Can you work these out from the model? Positions are in its coordinate system, mm. Face numbers are marked on the shaded views. A direction names the side the tool comes from. Coordinates: 2 decimals unless noted, no trailing zeros. Loops run counter-clockwise (first coordinate to the right, second up) from the corner with the lowest first, then second, coordinate; pieces in that order, holes last.
```python
from build123d import *

# Parameters (mm, degrees)
SKETCH1_W                  = 50
SKETCH1_H                  = 56
BOSS_EXTRUDE1_DEPTH        = 10
SKETCH2_R                  = 5.5
CUT_EXTRUDE1_DEPTH         = 59.172158289
CUT_EXTRUDE2_DEPTH         = 40.5
FILLET1_R                  = 3.6
F_5_2_5_2_DIAMETER_HOLE1_D = 5.2
SKETCH7_W                  = 3
SKETCH7_H                  = 29.868058684
CUT_EXTRUDE3_DEPTH         = 5
SKETCH8_W                  = 5.3
SKETCH8_H                  = 10
CUT_EXTRUDE4_DEPTH         = 15
CUT_EXTRUDE5_DEPTH         = 46.923850013
SKETCH10_W                 = 6.3
SKETCH10_H                 = 11
CUT_EXTRUDE6_DEPTH         = 10
CHAMFER1_SIZE              = 2
CHAMFER2_SIZE              = 2
SKETCH12_W                 = 1.5
SKETCH12_H                 = 0.75
SKETCH12_W_2               = 0.75
SKETCH12_H_2               = 1.5
CUT_EXTRUDE_THIN1_DEPTH    = 0.5


with BuildPart() as part:
    # Sketch1 → Boss-Extrude1 (new body)
    with BuildSketch(Plane(origin=(0, 0, 0), x_dir=(1, 0, 0), z_dir=(0, 1, 0))):
        Rectangle(SKETCH1_W, SKETCH1_H)
    extrude(amount=BOSS_EXTRUDE1_DEPTH)

    # Sketch2 → Cut-Extrude1 (cut, through all)
    with BuildSketch(Plane.ZY.offset(25)):
        with Locations((-13, 10)):
            Circle(SKETCH2_R)
        with Locations((2.468847143, 10)):
            Circle(SKETCH2_R)
    extrude(amount=-CUT_EXTRUDE1_DEPTH, mode=Mode.SUBTRACT)

    # Sketch3 → Cut-Extrude2 (cut)
    with BuildSketch(Plane.ZY.offset(25)):
        with BuildLine():
            Line((-20.736152857, 16.807330276), (-20.736152857, 2.265))
            Line((-20.736152857, 2.265), (-13.001152857, 2.265))
            ThreePointArc((-13.001152857, 2.265), (-10.106686283, 2.826974958), (-7.632806065, 4.431240918))
            ThreePointArc((-7.632806065, 4.431240918), (-5.266152857, 5.386235298), (-2.899499649, 4.431240918))
            ThreePointArc((-2.899499649, 4.431240918), (10.132273811, 8.950182537), (-1.204091668, 16.807330276))
            Line((-1.204091668, 16.807330276), (-20.736152857, 16.807330276))
        make_face()
    extrude(amount=-CUT_EXTRUDE2_DEPTH, mode=Mode.SUBTRACT)

    # Fillet1
    fillet1_edges = [part.edges().sort_by_distance(p)[0] for p in [
        (-4.75, 2.265, -20.736152857),
    ]]
    fillet(fillet1_edges, radius=FILLET1_R)

    # Ø5.2 (5.2) Diameter Hole1 (through all)
    with Locations(Plane(origin=(0, 10, 0), x_dir=(1, 0, 0), z_dir=(0, 1, 0))):
        with Locations((2.378026924, 24.5), (21.342971966, -14.059218087), (-21.342971966, -14.059218087)):
            Hole(F_5_2_5_2_DIAMETER_HOLE1_D / 2)

    # Sketch7 → Cut-Extrude3 (cut)
    with BuildSketch(Plane(origin=(0, 10, 0), x_dir=(1, 0, 0), z_dir=(0, 1, 0))):
        with Locations((16.76197527, 27.631709684)):
            Rectangle(SKETCH7_W, SKETCH7_H)
    extrude(amount=-CUT_EXTRUDE3_DEPTH, mode=Mode.SUBTRACT)

    # Sketch8 → Cut-Extrude4 (cut)
    with BuildSketch(Plane.ZY.offset(25)):
        with Locations((22.329609043, 10)):
            Rectangle(SKETCH8_W, SKETCH8_H)
    extrude(amount=-CUT_EXTRUDE4_DEPTH, mode=Mode.SUBTRACT)

    # Sketch9 → Cut-Extrude5 (cut, through all)
    with BuildSketch(Plane.ZY.offset(10)):
        with BuildLine():
            Line((24.329609043, 12.5), (24.329609043, 7.5))
            ThreePointArc((24.329609043, 7.5), (22.329609043, 5.5), (20.329609043, 7.5))
            Line((20.329609043, 7.5), (20.329609043, 12.5))
            ThreePointArc((20.329609043, 12.5), (22.329609043, 14.5), (24.329609043, 12.5))
        make_face()
    extrude(amount=-CUT_EXTRUDE5_DEPTH, mode=Mode.SUBTRACT)

    # Sketch10 → Cut-Extrude6 (cut)
    with BuildSketch(Plane.ZY.offset(25)):
        with Locations((22.329609043, 10)):
            Rectangle(SKETCH10_W, SKETCH10_H)
    extrude(amount=-CUT_EXTRUDE6_DEPTH, mode=Mode.SUBTRACT)

    # Chamfer1
    chamfer1_edges = [part.edges().sort_by_distance(p)[0] for p in [
        (-25, 7.25, 25.479609043),
        (-25, 7.25, 19.179609043),
        (-25, 4.5, 22.329609043),
        (-25, 7.9325, -20.736152857),
        (-25, 2.826974958, -10.106686283),
        (-25, 5.386235298, -5.266152857),
        (-25, 2.881208409, 5.494244849),
        (-25, 2.265, -15.068652857),
        (-25, 3.319415588, -19.681737269),
    ]]
    chamfer(chamfer1_edges, length=CHAMFER1_SIZE)

    # Chamfer2
    chamfer2_edges = [part.edges().sort_by_distance(p)[0] for p in [
        (25, 8.75, 24.329609043),
        (25, 8.75, 20.329609043),
        (25, 5.5, 22.329609043),
        (25, 4.5, -13),
        (25, 4.5, 2.468847143),
    ]]
    chamfer(chamfer2_edges, length=CHAMFER2_SIZE)

    # Sketch12 → Cut-Extrude-Thin1 (cut)
    with BuildSketch(Plane(origin=(0, 5, 0), x_dir=(1, 0, 0), z_dir=(0, 1, 0))):
        with Locations((-12.5, -22.329609043)):
            Rectangle(SKETCH12_W, SKETCH12_H)
        with Locations((-12.5, -22.329609043)):
            Rectangle(SKETCH12_W_2, SKETCH12_H_2)
    extrude(amount=-CUT_EXTRUDE_THIN1_DEPTH, mode=Mode.SUBTRACT)


solid = part.part
```
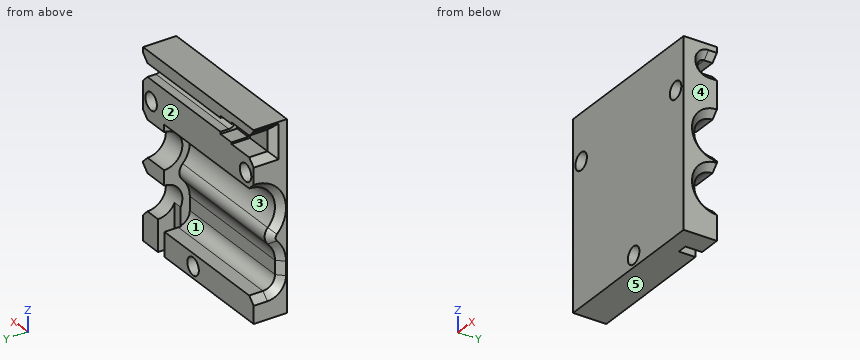
(1) Which directions (+Z, -Z, +X, -X, +Y, -Y) give clear straight access to the entire face, cutting with the end or side of a thin tool? Please do the marked faces 1 and 2.
Check values:
face 1: -X, +Y
face 2: +Z, -Z, +X, -X, +Y
(2) I want a section at A-A on x = -18. Write out the boundary of the cut face in (y, z) (1 decimal), then the cut area to 3 significant figures.
Check values:
outline: (0, -28) - (10, -28) - (10, -20.7) - (5.9, -20.7) arc R3.6 cw to (2.3, -17.1) - (2.3, -13) arc R7.7 cw to (4.4, -7.6) arc R3.4 ccw to (4.4, -2.9) arc R7.7 cw to (10, 10.2) - (10, 19.2) - (4.5, 19.2) - (4.5, 25.5) - (10, 25.5) - (10, 28) - (0, 28) - close
area: 322 mm2
(3) I want a section at B-B on x = -5.5. Write out the boundary of the cut face in (y, z) (1 decimal), then the cut area to 3 significant figures.
Check values:
outline: (0, -28) - (10, -28) - (10, -20.7) - (5.9, -20.7) arc R3.6 cw to (2.3, -17.1) - (2.3, -13) arc R7.7 cw to (4.4, -7.6) arc R3.4 ccw to (4.4, -2.9) arc R7.7 cw to (10, 10.2) - (10, 20.3) - (7.5, 20.3) arc R2 cw to (7.5, 24.3) - (10, 24.3) - (10, 28) - (0, 28) - close
area: 341 mm2
(4) If we mould it in two halves opening along Z, with no side actions, what happens to the marked faces 3, 4 and 5? For each: released by +Z, released by -Z, zero draft, split by the parting line, or undercut.
Check values:
face 3: undercut
face 4: zero draft
face 5: released by -Z
(5) If I drill on probe 1 along X at (y, z) = (7, -24.5); probe 2 along Z at (x, y) = (7, 9.75); probe 3 along Z at (x, y) = (-9, 6), over which ranges is the centre line in solid material (lowest first)?
Check values:
probe 1: x = -25 to -0.22, 4.98 to 15.26, 18.26 to 25
probe 2: z = -28 to -20.74, 10.2 to 20.33, 24.33 to 28
probe 3: z = -28 to -20.74, 9.09 to 21.01, 23.65 to 28
(6) I'm going to push flat-ended pins straight in: pin 1 (12 mm diameter, centred on x = -4, z = -7, fed in from +Y); pin 2 (1.5 mm diameter, centred on x = 16.5, z = -10.5, fed in from +Y); pin 3 (1 mm diameter, centred on y = 7.5, z = 5.5, fed in from -X); pin 4 (1.2 mm diameter, centred on x = -13.5, z = -16, fed in from +Y) (3 decimals). Where does each tip first touch, or does it pass through?
Check values:
pin 1: stops at y = 5.39
pin 2: stops at y = 5.56
pin 3: passes through
pin 4: stops at y = 2.265
